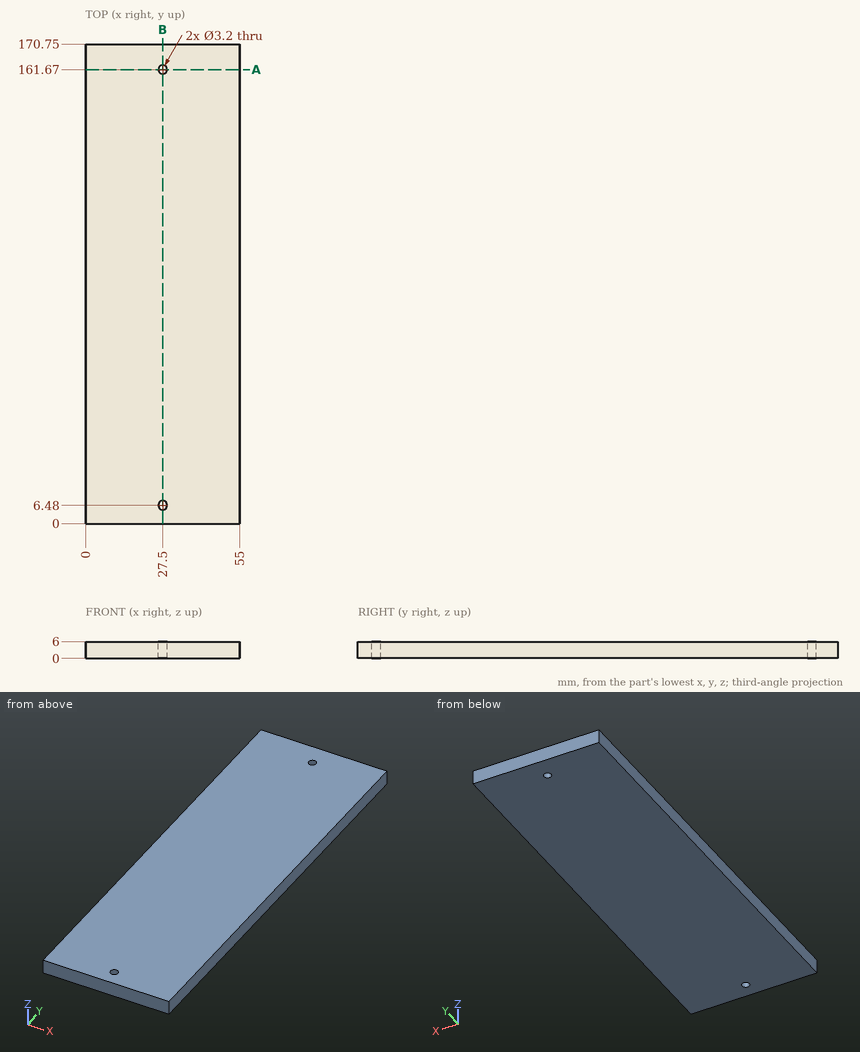
Input: dimensioned drawing with shaded views. Units: mm. Origin: part minimum x, y, z. Coordinates: 2 decimals unless noted, no trailing zeros. Loops run counter-clockwise (first coordinate to the right, second up) from the corner with the lowest first, then second, coordinate; pieces in that order, holes last. Notation, with made-up numbers: M 77.25,-3 L 95.25,-3 A23 cw 95.25,19 Z; hole C 78,-34 d9. An arc over 180 degrees is marked long. Use a Markdown table: item, result. Add a question column.
Q1. Section query A-A, the plane y = 161.67. Return loops of the section in (x, z).
Q2. Section query B-B, the plane x = 27.5. Return loops of the section in (y, z), and give its area (3 significant figures).
Q3. Material intervals for L1, parallel to Y at x = 27.5, z = 2.4; L2, parallel to X at y = 161.67, z = 2.3, sorted ascending.
Result:
| question | item | result |
|---|---|---|
| 1 | outline | M 0,0 L 25.9,0 L 25.9,6 L 0,6 Z; M 29.1,0 L 55,0 L 55,6 L 29.1,6 Z |
| 2 | outline | M 0,0 L 4.88,0 L 4.88,6 L 0,6 Z; M 8.08,0 L 160.07,0 L 160.07,6 L 8.08,6 Z; M 163.27,0 L 170.75,0 L 170.75,6 L 163.27,6 Z |
| 2 | area | 986 mm2 |
| 3 | L1 | y = 0 to 4.88, 8.08 to 160.07, 163.27 to 170.75 |
| 3 | L2 | x = 0 to 25.9, 29.1 to 55 |
